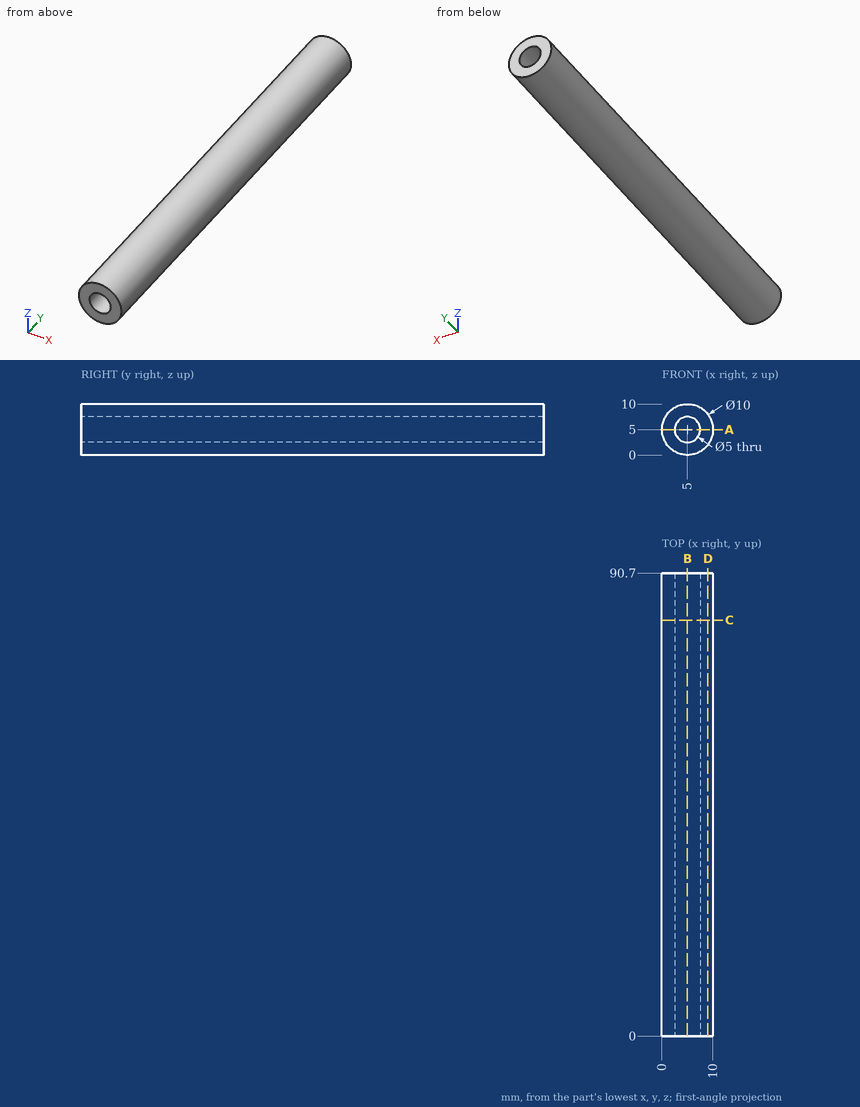
For this review, use the dimensioned drawing (mm, ordinates from the lowest corner) and the shaded views. Round coordinates to 2 decimals unless told otherwise and drop trailing zeros. Order: outer loops, then holes, each group sorted by start corner. A loop starts at its lowest first (then second) coordinate and runs counter-clockwise, first axis right, second up. Notation, with made-up numbers: (14.25, 41) -> (30.25, 41) arc R22 cw to (30.25, 49) -> close; hole circle Ø9 at (78, 78). An arc over 180 degrees is marked (long way). One line per item, written item: value. Start each with the question number.
Q1. Take a section at C-C (y = 81.5). Write out the cut boundary in (x, z), and give its area (3 significant figures).
Q2. Take a section at D-D (x = 9). Write out the cut boundary in (y, z), and give its area (3 significant figures).
Q3. Clearance check with flat-ended pins moving along their axes: pin 1 Ø1 at (y, z) = (63.5, 6) entering from +X; pin 2 Ø2 at (y, z) = (21, 6.5) entering from -X; pin 3 Ø4.5 at (x, z) = (5, 5) entering from +Y. State where each tip first meets the part, or that it passes through.
Q4. Take a section at B-B (x = 5). Write out the cut boundary in (y, z).
Q5. Take a section at A-A (z = 5). Write out the cut boundary in (x, y).
Q6. Wall thickness on line 1 (Z direction, x = 5, y = 37); line 2 (Z direction, x = 7, y = 84.5): over which ranges is each line inside the solid? List them lowest first.
Reported:
1. outline: circle Ø10 at (5, 5); hole circle Ø5 at (5, 5)
1. area: 58.9 mm2
2. outline: (0, 2) -> (90.7, 2) -> (90.7, 8) -> (0, 8) -> close
2. area: 544 mm2
3. pin 1: stops at x = 9.97
3. pin 2: stops at x = 0.03
3. pin 3: passes through
4. outline: (0, 0) -> (90.7, 0) -> (90.7, 2.5) -> (0, 2.5) -> close; (0, 7.5) -> (90.7, 7.5) -> (90.7, 10) -> (0, 10) -> close
5. outline: (0, 0) -> (2.5, 0) -> (2.5, 90.7) -> (0, 90.7) -> close; (7.5, 0) -> (10, 0) -> (10, 90.7) -> (7.5, 90.7) -> close
6. line 1: z = 0 to 2.5, 7.5 to 10
6. line 2: z = 0.42 to 3.5, 6.5 to 9.58
